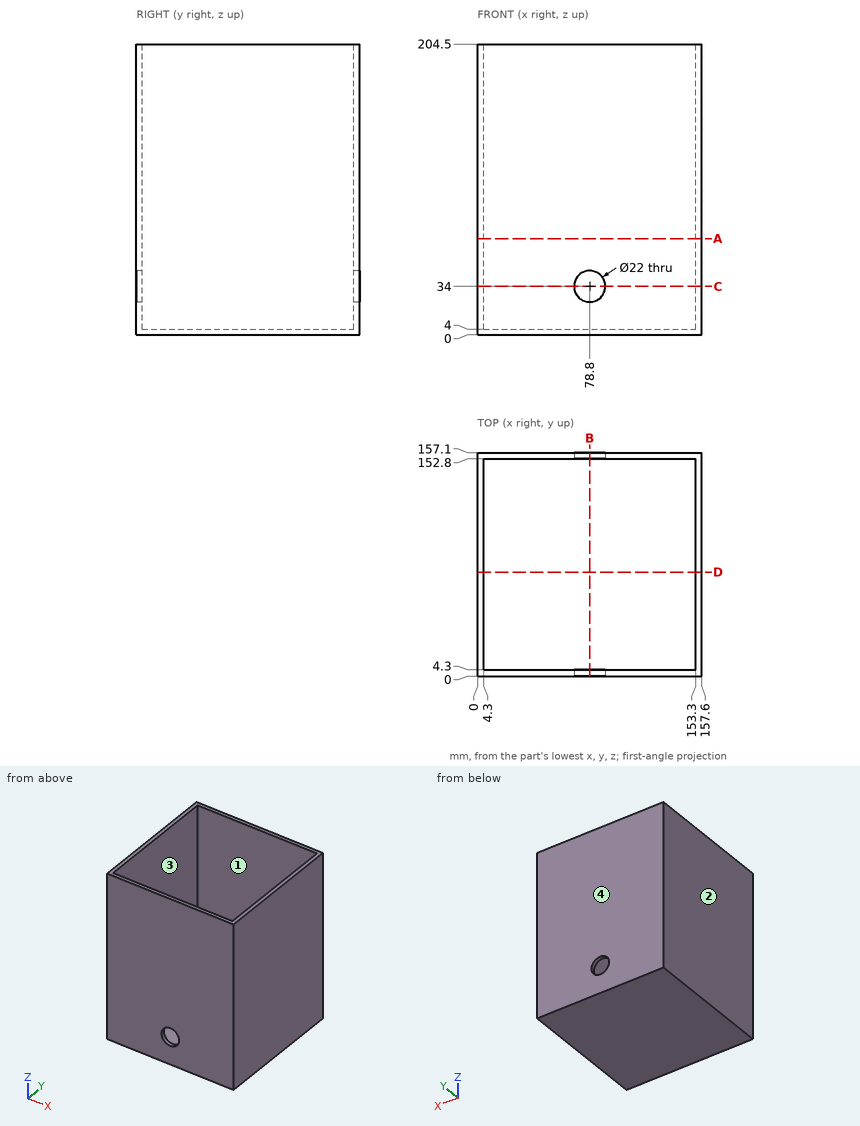
Part print with two shaded views. Sizes in mm from the minimum x, y, z corner. Round coordinates to 2 decimals unless told otherwise and drop trailing zeros. Order: outer loops, then holes, each group sorted by start corner. A loop starts at its lowest first (then second) coordinate and runs counter-clockwise, first axis right, second up. Notation, with made-up numbers: M 86,11.25 L 101,11.25 A26 cw 101,40.25 Z; hole C -5,7 d6. An arc over 180 degrees is marked long. Put each result on its own line as item: value. Start each with the question number.
1. Slice it at A-A on z = 67.5. List the corners of the cut face in (x, y), then the cut area to 3 significant figures.
2. Two-plate mould, pull along Y, no slides. Class the marked faces 1, 2, 3 and 4: +Y half, -Y half, draft (parallel to the pull), parting line (faces both ways), or undercut.
3. Drop a flat-ended pin along its axis: pin 1 (4 mm diameter, centred on x = 35.5, y = 96.5, fed in from +Z). Give the stop position or say it passes through.
4. Slice it at B-B on x = 78.8. List the corners of the cut face in (y, z), then the cut area to 3 significant figures.
5. Slice it at C-C on z = 34. List the corners of the cut face in (x, y).
6. Slice it at D-D on y = 73. List the corners of the cut face in (x, z).
7. Drill centre lines: probe 1 along Z at (x, y) = (78, 154); probe 2 along Y at (x, z) = (35.5, 100); probe 3 along X at (y, z) = (115.5, 18.5). Where is each one in solid material? Low to high. Write a range as [from, to].
Findings:
1. outline: M 0,0 L 157.6,0 L 157.6,157.1 L 0,157.1 Z; hole M 4.3,4.3 L 153.3,4.3 L 153.3,152.8 L 4.3,152.8 Z
1. area: 2,630 mm2
2. face 1: undercut
2. face 2: draft
2. face 3: undercut
2. face 4: +Y half
3. pin 1: z = 4
4. outline: M 0,0 L 157.1,0 L 157.1,23 L 152.8,23 L 152.8,4 L 4.3,4 L 4.3,23 L 0,23 Z; M 0,45 L 4.3,45 L 4.3,204.5 L 0,204.5 Z; M 152.8,45 L 157.1,45 L 157.1,204.5 L 152.8,204.5 Z
4. area: 2,160 mm2
5. outline: M 0,0 L 67.8,0 L 67.8,4.3 L 4.3,4.3 L 4.3,152.8 L 67.8,152.8 L 67.8,157.1 L 0,157.1 Z; M 89.8,0 L 157.6,0 L 157.6,157.1 L 89.8,157.1 L 89.8,152.8 L 153.3,152.8 L 153.3,4.3 L 89.8,4.3 Z
6. outline: M 0,0 L 157.6,0 L 157.6,204.5 L 153.3,204.5 L 153.3,4 L 4.3,4 L 4.3,204.5 L 0,204.5 Z
7. probe 1: [0, 23.03], [44.97, 204.5]
7. probe 2: [0, 4.3], [152.8, 157.1]
7. probe 3: [0, 4.3], [153.3, 157.6]
